Geometry: final body of the model. Coordinates: model frame, mm. Coordinates: 2 decimals unless noted, no trailing zeros. Write each loop counter-clockwise with the first axis right and the second up, starting at its lowest first coordinate (ties: lowest second). Pieces come first, ordered by that corner, then holes.
from build123d import *

# Parameters (mm, degrees)
F0_W     = 609.6
F0_H     = 4.916123
F0_H_2   = 203.2
F1_DEPTH = 218.44


with BuildPart() as f1:
    # F0 (on Front) → F1 (new body)
    with BuildSketch(Plane.XZ):
        with Locations((0, -104.058061)):
            Rectangle(F0_W, F0_H)
        Rectangle(F0_W, F0_H_2)
        Polygon((-304.8, 101.6), (304.8, 101.6), (304.8, 106.516123), (-276.664647, 106.516123), align=None)
        Polygon((-304.8, 106.516123), (-304.8, 101.6), (-276.664647, 106.516123), align=None)
        Polygon((-276.664647, 106.516123), (304.8, 106.516123), (304.8, 208.116123), align=None)
    extrude(amount=F1_DEPTH)


solid = f1.part
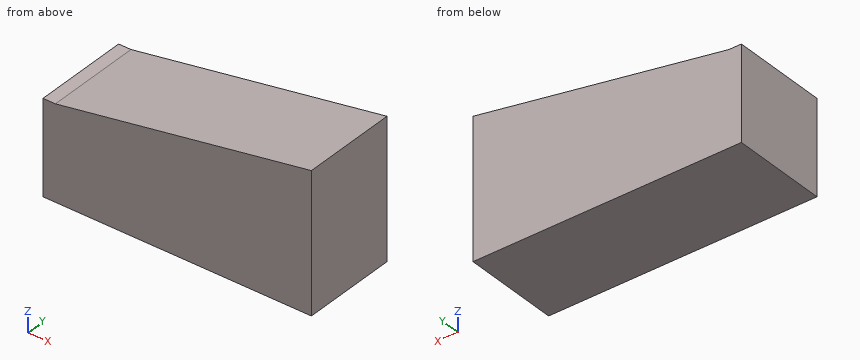
Item 1: Section A-A, the plane y = -175. Output: boundary loops of the cut face in (x, z), plus the area to 3 significant figures.
Derived:
outline: (-304.8, -106.52) - (304.8, -106.52) - (304.8, 208.12) - (-276.66, 106.52) - (-304.8, 106.52) - close
area: 159,000 mm2
Item 2: Section C-C, the plane z = 149.5. Output: boundary loops of the cut face in (x, y).
Derived:
outline: (-30.66, -218.44) - (304.8, -218.44) - (304.8, 0) - (-30.66, 0) - close
Item 3: Section B-B, the plane x = -199.5. Output: boundary loops of the cut face in (y, z).
Derived:
outline: (-218.44, -106.52) - (0, -106.52) - (0, 120) - (-218.44, 120) - close
Item 4: Pin query (flat end, axial travel): pin 1 (6 mm diameter, centred on x = 99, z = 75, fed in from +Y). Return the tip coordinate at first contact, or that it passes through.
Derived:
pin 1: stops at y = 0
Item 5: Material intervals for probe 1 along Z at (x, y) = (104.5, -34.5); probe 2 along Z at (x, y) = (248.5, -209), sorted ascending.
Derived:
probe 1: z = -106.52 to 173.12
probe 2: z = -106.52 to 198.28
